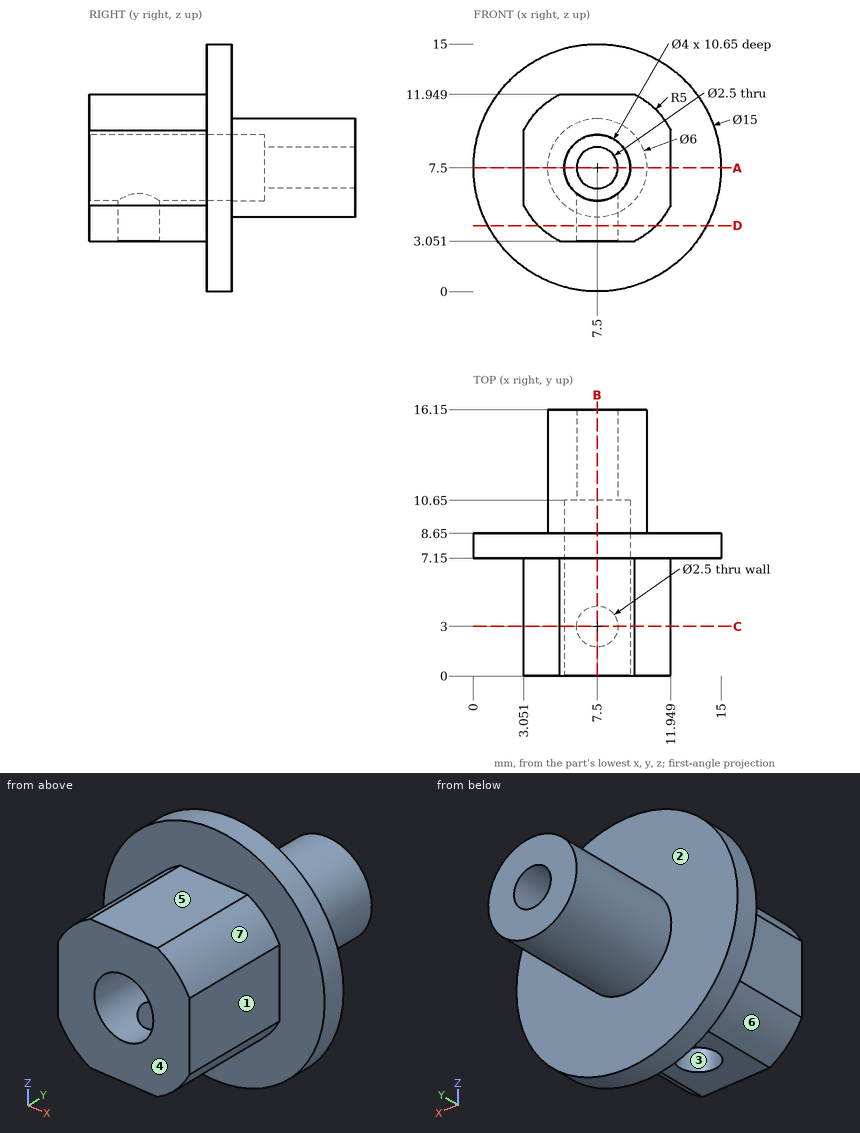
Study the drawing (mm; zero at the part's minimum x, y, z) and answer. A direction names the side the tool comes from. Round coordinates to 2 decimals unless told otherwise and drop trailing zeros. Loops run counter-clockwise (first coordinate to the right, second up) from the corner with the lowest first, then second, coordinate; pieces in that order, holes last. Notation, with made-up numbers: (26.25, -21.75) -> (55.25, -21.75) arc R32 ccw to (55.25, 16.25) -> close; hole circle Ø10 at (79.5, 42). An arc over 180 degrees is marked (long way). One line per item, written item: value.
1) A cutting plane is placed at A-A (z = 7.5). Determine the outline of the cut face in (x, y), and give its area (3 significant figures).
Answer list:
outline: (0, 7.15) -> (3.05, 7.15) -> (3.05, 0) -> (5.5, 0) -> (5.5, 10.65) -> (6.25, 10.65) -> (6.25, 16.15) -> (4.5, 16.15) -> (4.5, 8.65) -> (0, 8.65) -> close; (8.75, 10.65) -> (9.5, 10.65) -> (9.5, 0) -> (11.95, 0) -> (11.95, 7.15) -> (15, 7.15) -> (15, 8.65) -> (10.5, 8.65) -> (10.5, 16.15) -> (8.75, 16.15) -> close
area: 74.8 mm²
2) Consider L1, parallel to Y at x = 7.5, z = 5.1; L2, parallel to X at y = 4.25, z = 7.5. Determine where each line is inside the solid, lowest interval first. Write a range as [from, to].
Answer list:
L1: y = [0, 1.75], [4.25, 16.15]
L2: x = [3.05, 5.5], [9.5, 11.95]
3) Flat-ended cylindrical pins translate along their axes: P1, Ø3.5, axis at y = 4, z = 7, coming from the -X side; P2, Ø1.5, axis at x = 7.5, z = 7.5, coming from the -Y side; P3, Ø5, axis at y = 3.5, z = 7, coming from the +X side; P4, Ø1, axis at x = 3.5, z = 8, coming from the +Y side. Find the tip coordinate at first contact, or state that the pin passes through.
Answer list:
P1: stops at x = 3.05
P2: passes through
P3: stops at x = 11.95
P4: stops at y = 8.65
4) A cutting plane is placed at C-C (y = 3). Determine the outline of the cut face in (x, z), and give its area (3 significant figures).
Answer list:
outline: (3.05, 5.22) arc R5 ccw to (5.22, 3.05) -> (6.25, 3.05) -> (6.25, 5.94) arc R2 cw (long way) to (8.75, 5.94) -> (8.75, 3.05) -> (9.78, 3.05) arc R5 ccw to (11.95, 5.22) -> (11.95, 9.78) arc R5 ccw to (9.78, 11.95) -> (5.22, 11.95) arc R5 ccw to (3.05, 9.78) -> close
area: 52.7 mm²
5) The mould has two halves that part along Y. Classify the marked faces 1, 2, 3 and 4: pulls with the +Y half, pulls with the -Y half, needs draft (parallel to the pull), parting line crosses it, or undercut.
Answer list:
face 1: needs draft
face 2: pulls with the +Y half
face 3: undercut
face 4: pulls with the -Y half
6) For the marked faces 5, 6 and 7, determine the directions among +Z, -Z, +X, -X, +Y, -Y from which every point of the face is accessible in a straight line to the end or side of a thin tool.
Answer list:
face 5: +Z, +X, -X, -Y
face 6: -Z, -X, -Y
face 7: +Z, +X, -Y
7) A cutting plane is placed at D-D (z = 4). Determine the outline of the cut face in (x, y).
Answer list:
outline: (0.87, 7.15) -> (3.93, 7.15) -> (3.93, 0) -> (11.07, 0) -> (11.07, 7.15) -> (14.13, 7.15) -> (14.13, 8.65) -> (0.87, 8.65) -> close; hole circle Ø2.5 at (7.5, 3)
8) A cutting plane is placed at B-B (x = 7.5). Determine the outline of the cut face in (y, z).
Answer list:
outline: (0, 3.05) -> (1.75, 3.05) -> (1.75, 5.5) -> (0, 5.5) -> close; (0, 9.5) -> (10.65, 9.5) -> (10.65, 8.75) -> (16.15, 8.75) -> (16.15, 10.5) -> (8.65, 10.5) -> (8.65, 15) -> (7.15, 15) -> (7.15, 11.95) -> (0, 11.95) -> close; (4.25, 3.05) -> (7.15, 3.05) -> (7.15, 0) -> (8.65, 0) -> (8.65, 4.5) -> (16.15, 4.5) -> (16.15, 6.25) -> (10.65, 6.25) -> (10.65, 5.5) -> (4.25, 5.5) -> close
